```python
from build123d import *

# Parameters (mm, degrees)
BOX003_W     = 1
BOX003_H     = 2.7
BOX003_DEPTH = 10
BOX001_W     = 20.75
BOX001_H     = 5
BOX001_DEPTH = 10
BOX002_W     = 25.75
BOX002_H     = 5
BOX002_DEPTH = 10
BOX_W        = 31
BOX_H        = 16
BOX_DEPTH    = 10
FILLET_R     = 1


with BuildPart() as cube003:
    # Box003 → Box003 (new body)
    with BuildSketch(Plane(origin=(14, 18.3, 0), x_dir=(1, 0, 0), z_dir=(0, 0, 1))):
        with Locations((0.5, 1.35)):
            Rectangle(BOX003_W, BOX003_H)
    extrude(amount=BOX003_DEPTH)


with BuildPart() as cube001:
    # Box001 → Box001 (new body)
    with BuildSketch(Plane(origin=(0, 16, 0), x_dir=(1, 0, 0), z_dir=(0, 0, 1))):
        with Locations((10.375, 2.5)):
            Rectangle(BOX001_W, BOX001_H)
    extrude(amount=BOX001_DEPTH)


with BuildPart() as cube002:
    # Box002 → Box002 (new body)
    with BuildSketch(Plane(origin=(0, -5, 0), x_dir=(1, 0, 0), z_dir=(0, 0, 1))):
        with Locations((12.875, 2.5)):
            Rectangle(BOX002_W, BOX002_H)
    extrude(amount=BOX002_DEPTH)


with BuildPart() as fillet_body:
    # Box → Box (new body)
    with BuildSketch(Plane.XY):
        with Locations((15.5, 8)):
            Rectangle(BOX_W, BOX_H)
    extrude(amount=BOX_DEPTH)

    # Fusion: union Cube001, Cube002
    add(cube001.part)
    add(cube002.part)

    # Cut: cut Cube003
    add(cube003.part, mode=Mode.SUBTRACT)

    # Fillet
    fillet_edges = [fillet_body.edges().sort_by_distance(p)[0] for p in [
        (0, -5, 5),
        (25.75, -5, 5),
        (20.75, 21, 5),
        (0, 21, 5),
    ]]
    fillet(fillet_edges, radius=FILLET_R)


solid = fillet_body.part
```
For this review, take the finished solid that the model builds, in its own axes (mm). A direction names the side the tool comes from. Coordinates: 2 decimals unless noted, no trailing zeros. Loops run counter-clockwise (first coordinate to the right, second up) from the corner with the lowest first, then second, coordinate; pieces in that order, holes last.
1. Mouldability with a two-part tool opening along X and no side actions: class faces 4 (the flat face through (0, 8, 5)), 5 (the flat face through (14.5, 18.3, 4.9)), 6 (the flat face through (13, -5, 5)) as +X half, -X half, draft (parallel to the pull), parting line (faces both ways), or undercut.
2. Add section A-A, the plane z = 4. Give the boundary of the cut face in (x, y).
3. Add section C-C, the plane y = -1. Give the boundary of the cut face in (x, z).
4. Insertion check: P1, Ø4, axis at x = 29, z = 5.5, coming from the -Y side; P2, Ø2, axis at y = 18, z = 4.5, coming from the +X side; P3, Ø0.5, axis at x = 14.5, z = 5.5, coming from the +Y side; P4, Ø3, axis at y = -1, z = 7, coming from the +X side. Each pin has a flat end and moves straight along its axis. Give the tip position at first contact, or say it passes through.
5. Add section B-B, the plane x = 26.5. Give the boundary of the cut face in (y, z), then the cut area to 3 significant figures.
6. For line 1 (X direction, y = 17, z = 4); line 2 (X direction, y = -4, z = 2.5); line 3 (Y direction, x = 27, z = 4.5), list the stretches that pass through material, from the lowest coordinate up.
7. For faces 1 (the flat face through (20.75, 18, 5)), 2 (the flat face through (28, 0, 5)), 3 (the flat face through (14, 20, 5)), list the 3-axis set-ups (+Z, -Z, +X, -X, +Y, -Y) from which the entire face can be reached by the end or side of a thin tool; tool diameter is ignored.
Result:
1. face 4: -X half
1. face 5: undercut
1. face 6: draft
2. outline: (0, -4) arc R1 ccw to (1, -5) - (24.75, -5) arc R1 ccw to (25.75, -4) - (25.75, 0) - (31, 0) - (31, 16) - (20.75, 16) - (20.75, 20) arc R1 ccw to (19.75, 21) - (15, 21) - (15, 18.3) - (14, 18.3) - (14, 21) - (1, 21) arc R1 ccw to (0, 20) - close
3. outline: (0, 0) - (25.75, 0) - (25.75, 10) - (0, 10) - close
4. P1: stops at y = 0
4. P2: stops at x = 20.75
4. P3: stops at y = 18.3
4. P4: stops at x = 31
5. outline: (0, 0) - (16, 0) - (16, 10) - (0, 10) - close
5. area: 160 mm2
6. line 1: x = 0 to 20.75
6. line 2: x = 0 to 25.75
6. line 3: y = 0 to 16
7. face 1: +Z, -Z, +X, +Y
7. face 2: +Z, -Z, +X, -Y
7. face 3: +Z, -Z, +Y
